```python
from build123d import *

# Parameters (mm, degrees)
SKETCH_1_W                  = 125
SKETCH_1_H                  = 95
EXTRUDE_1_DEPTH             = 16
SKETCH_3_R                  = 1.75
CUT_EXTRUDE_1_DEPTH         = 158.816348963
CUT_EXTRUDE_2_DEPTH         = 13
CUT_EXTRUDE_3_DEPTH         = 158.816348963
EXTRUDE_4_DEPTH             = 80
HOLE_WIZARD_4_0_4_1_D       = 4
SKETCH_11_W                 = 42
SKETCH_11_H                 = 30
CUT_EXTRUDE_4_DEPTH         = 158.540470991
FILLET_4_R                  = 3
CHAMFER_1_SIZE              = 2.5
CHAMFER_1_SIZE2             = 3.535533906
HOLE_WIZARD_2_5_2_5_1_D     = 2.5
HOLE_WIZARD_2_5_2_5_1_DEPTH = 16
HOLE_WIZARD_2_5_2_5_1_TIP   = 0.751075774
CHAMFER_2_SIZE              = 1.5


with BuildPart() as part:
    # 草图1 → 凸台-拉伸1 (new body)
    with BuildSketch(Plane.XY):
        with Locations((62.5, 47.5)):
            Rectangle(SKETCH_1_W, SKETCH_1_H)
    extrude(amount=EXTRUDE_1_DEPTH)

    # 草图3 → 切除-拉伸1 (cut, through all)
    with BuildSketch(Plane.XY.offset(16)):
        with Locations((26.91, 90)):
            Circle(SKETCH_3_R)
        with Locations((26.91, 20.71)):
            Circle(SKETCH_3_R)
        with Locations((120, 90)):
            Circle(SKETCH_3_R)
        with Locations((120, 20.71)):
            Circle(SKETCH_3_R)
    extrude(amount=-CUT_EXTRUDE_1_DEPTH, mode=Mode.SUBTRACT)

    # 草图4 → 切除-拉伸2 (cut)
    with BuildSketch(Plane.XY.offset(16)):
        Polygon((33, 95), (33, 86.8), (17, 86.8), (17, 25.71), (33, 25.71), (33, 0), (113, 0), (113, 25.71), (125, 25.71), (125, 86.8), (113, 86.8), (113, 95), align=None)
    extrude(amount=-CUT_EXTRUDE_2_DEPTH, mode=Mode.SUBTRACT)

    # 草图5 → 切除-拉伸3 (cut, through all)
    with BuildSketch(Plane(origin=(125, 0, 0), x_dir=(0, 0, -1), z_dir=(1, 0, 0))):
        Polygon((-16, 0), (0, 16), (0, 0), align=None)
    extrude(amount=-CUT_EXTRUDE_3_DEPTH, mode=Mode.SUBTRACT)

    # 草图8 → 凸台-拉伸4 (add)
    with BuildSketch(Plane(origin=(33, 0, 0), x_dir=(0, 0, -1), z_dir=(1, 0, 0))):
        Polygon((-16, 0), (-3, 13), (-3, 18.656854249), (-16, 5.656854249), align=None)
    extrude(amount=EXTRUDE_4_DEPTH)

    # Ø4.0 (4) 直径孔1 (through all)
    with Locations(Plane(origin=(0, 10.828427125, 10.828427125), x_dir=(1, 0, 0), z_dir=(0, 0.7071067811865476, 0.7071067811865476))):
        with Locations((43, 1.186291501), (103, 1.186291501)):
            Hole(HOLE_WIZARD_4_0_4_1_D / 2)

    # 草图11 → 切除-拉伸4 (cut, through all)
    with BuildSketch(Plane.XY.offset(3)):
        with Locations((63.91, 50)):
            Rectangle(SKETCH_11_W, SKETCH_11_H)
    extrude(amount=-CUT_EXTRUDE_4_DEPTH, mode=Mode.SUBTRACT)

    # 圆角4
    fillet_4_edges = [part.edges().sort_by_distance(p)[0] for p in [
        (25, 86.8, 3),
        (113, 90.9, 3),
        (119, 86.8, 3),
        (119, 25.71, 3),
        (25, 25.71, 3),
        (33, 90.9, 3),
    ]]
    fillet(fillet_4_edges, radius=FILLET_4_R)

    # 倒角1
    chamfer_1_edges = [part.edges().sort_by_distance(p)[0] for p in [
        (62.5, 0, 16),
    ]]
    chamfer_1_side = [part.faces().sort_by_distance(p)[0] for p in [
        (62.405862979, 7.992479485, 8.007520515),
    ]]
    chamfer(chamfer_1_edges, length=CHAMFER_1_SIZE, length2=CHAMFER_1_SIZE2, reference=chamfer_1_side[0])

    # Ø2.5 (2.5) 直径孔1
    with Locations(Plane.ZY):
        with Locations((8, 83), (8, 53), (8, 23)):
            Hole(HOLE_WIZARD_2_5_2_5_1_D / 2, depth=HOLE_WIZARD_2_5_2_5_1_DEPTH)
            with Locations((0, 0, -(HOLE_WIZARD_2_5_2_5_1_DEPTH + HOLE_WIZARD_2_5_2_5_1_TIP / 2))):  # 118° drill point
                Cone(0, HOLE_WIZARD_2_5_2_5_1_D / 2, HOLE_WIZARD_2_5_2_5_1_TIP, mode=Mode.SUBTRACT)

    # 倒角2
    chamfer_2_edges = [part.edges().sort_by_distance(p)[0] for p in [
        (62.5, 95, 0),
    ]]
    chamfer(chamfer_2_edges, length=CHAMFER_2_SIZE)


solid = part.part
```
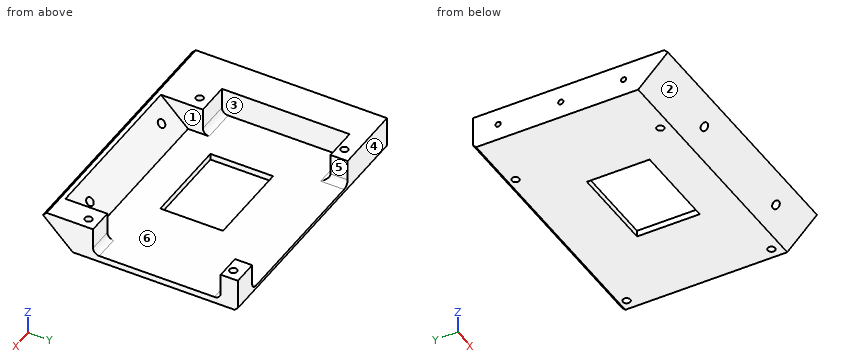
The model under review builds one solid part; all positions refer to its coordinate system, in mm. Face numbers are marked on the shaded views. A direction names the side the tool comes from. Round coordinates to 2 decimals unless told otherwise and drop trailing zeros. Order: outer loops, then holes, each group sorted by start corner. A loop starts at its lowest first (then second) coordinate and runs counter-clockwise, first axis right, second up.
(1) Take a section at A-A, the plane y = 61.5. State the section outline as (x, z) points.
Working result:
outline: (0, 0) - (42.91, 0) - (42.91, 3) - (17, 3) - (17, 16) - (0, 16) - close; (84.91, 0) - (125, 0) - (125, 3) - (84.91, 3) - close
(2) Tool access review of the marked faces 4, 5 and 6: name each direction out of +Z, -Z, +X, -X, +Y, -Y from which nothing blocks a thin tool from reaching the whole face with its end or side.
Working result:
face 4: +Z, -Z, +X, -X, +Y
face 5: +Z, +Y
face 6: +Z
(3) For P1, Ø8, axis at x = 120, z = 10, coming from the -Y side; P2, Ø2, axis at y = 83, z = 8, coming from the -X side; P3, Ø2, axis at x = 19.5, y = 77, coming from the +Z side, all flat-tipped, find the tip position at first contact; note any pin that passes through.
Working result:
P1: stops at y = 2
P2: stops at x = 16.15
P3: stops at z = 3
(4) Take a section at D-D, the plane x = 50.5. State the section outline as (y, z) points, plus the area to 3 significant figures.
Working result:
outline: (1.77, 14.23) - (16, 0) - (35, 0) - (35, 3) - (18.66, 3) - (5.66, 16) - (3.54, 16) - close; (65, 0) - (93.5, 0) - (95, 1.5) - (95, 3) - (65, 3) - close
area: 221 mm2
(5) Wall thickness on L1, parallel to Y at x = 120, z = 9.5; L2, parallel to Y at x = 11.5, z = 8; L3, parallel to X at y = 9, z = 14.25: over which ranges is each line inside the solid? List them lowest first.
Working result:
L1: y = 6.5 to 18.96, 22.46 to 25.71, 86.8 to 88.25, 91.75 to 95
L2: y = 8 to 21.75, 24.25 to 51.75, 54.25 to 81.75, 84.25 to 95
L3: x = 0 to 33, 113 to 125
(6) Mouldability with a two-part tool opening along X and no side actions: class the marked faces 1, 2 and 3 as released by +X, released by -X, zero draft, split by the parting line, or undercut.
Working result:
face 1: undercut
face 2: zero draft
face 3: released by +X
(7) Take a section at B-B, the plane x = 26.91. State the section outline as (y, z) points.
Working result:
outline: (1.77, 14.23) - (16, 0) - (18.96, 0) - (18.96, 16) - (3.54, 16) - close; (22.46, 0) - (88.25, 0) - (88.25, 16) - (86.8, 16) - (86.8, 6) arc R3 cw to (83.8, 3) - (28.71, 3) arc R3 cw to (25.71, 6) - (25.71, 16) - (22.46, 16) - close; (91.75, 0) - (93.5, 0) - (95, 1.5) - (95, 16) - (91.75, 16) - close
(8) Take a section at C-C, the plane y = 90. State the section outline as (x, z) points.
Working result:
outline: (0, 0) - (25.16, 0) - (25.16, 16) - (0, 16) - close; (28.66, 0) - (118.25, 0) - (118.25, 16) - (113, 16) - (113, 6) arc R3 cw to (110, 3) - (36, 3) arc R3 cw to (33, 6) - (33, 16) - (28.66, 16) - close; (121.75, 0) - (125, 0) - (125, 16) - (121.75, 16) - close
